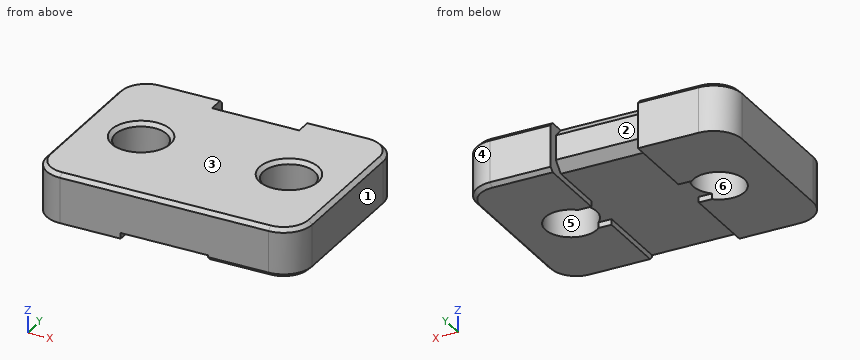
Autodesk Fusion 360 part; units mm, degrees
sketch "Sketch1" plane through (0, 0, 0) normal (0, 0, 1) x (1, 0, 0) in component "[a]_z_belt_clip_upper_x4"
  line L0 (14, -10) -> (-14, -10)
  line L1 (-14, -10) -> (-14, 10)
  line L2 (-14, 10) -> (14, 10)
  line L3 (14, 10) -> (14, -10)
  line L4 (14, -10) -> (-14, 10) construction
  line L5 (-14, -10) -> (14, 10) construction
  circle A0 centre (-7.8, 0) radius 2.7
  circle A1 centre (7.8, 0) radius 2.7
  dimension "d4" = 28
  dimension "d5" = 20
  dimension "d6" = 5.4
  dimension "d7" = 5.4
  dimension "d8" = 6.2
  dimension "d9" = 6.2
extrude "Extrude1" add sketch "Sketch1" along normal mid plane 5.2 in component "[a]_z_belt_clip_upper_x4"
fillet "Fillet1" radius 3 4 edges at (14, -10, 0) (14, 10, 0) (-14, -10, 0) (-14, 10, 0) in component "[a]_z_belt_clip_upper_x4"
sketch "Sketch2" plane through (0, 0, 2.6) normal (0, 0, 1) x (-1, 0, 0) in component "[a]_z_belt_clip_upper_x4"
  arc A0 (11, -10) -> (14, -7) centre (11, -7) ccw
  line L0 (14, -7) -> (14, 7)
  arc A1 (14, 7) -> (11, 10) centre (11, 7) ccw
  line L1 (11, 10) -> (-11, 10)
  arc A2 (-11, 10) -> (-14, 7) centre (-11, 7) ccw
  line L2 (-14, 7) -> (-14, -7)
  arc A3 (-14, -7) -> (-11, -10) centre (-11, -7) ccw
  line L3 (-11, -10) -> (11, -10)
  circle A4 centre (-7.8, 0) radius 2.7
  circle A5 centre (7.8, 0) radius 2.7
  line L4 (-4.6, -9) -> (4.6, -9)
  line L5 (4.6, -9) -> (4.6, -10)
  line L6 (4.6, -10) -> (-4.6, -10)
  line L7 (-4.6, -10) -> (-4.6, -9)
  line L8 (-4.6, -9) -> (4.6, -10) construction
  line L9 (4.6, -9) -> (-4.6, -10) construction
  line L10 (0, 0) -> (0, -20) construction
  point P0 (0, -9.5)
  dimension "d14" = 9.2
  dimension "d15" = 1
extrude "Extrude2" cut sketch "Sketch2" along normal through all and the other way through all contours L3 L4 L5 L6 L7 in component "[a]_z_belt_clip_upper_x4"
sketch "Sketch3" plane through (0, 0, -2.6) normal (0, 0, -1) x (1, 0, 0) in component "[a]_z_belt_clip_upper_x4"
  line L0 (4.6, -9) -> (4.6, -10)
  line L1 (4.6, -10) -> (11, -10)
  arc A0 (11, -10) -> (14, -7) centre (11, -7) ccw
  line L2 (14, -7) -> (14, 7)
  arc A1 (14, 7) -> (11, 10) centre (11, 7) ccw
  line L3 (11, 10) -> (-11, 10)
  arc A2 (-11, 10) -> (-14, 7) centre (-11, 7) ccw
  line L4 (-14, 7) -> (-14, -7)
  arc A3 (-14, -7) -> (-11, -10) centre (-11, -7) ccw
  line L5 (-11, -10) -> (-4.6, -10)
  line L6 (-4.6, -10) -> (-4.6, -9)
  line L7 (-4.6, -9) -> (4.6, -9)
  circle A4 centre (7.8, 0) radius 2.7
  circle A5 centre (-7.8, 0) radius 2.7
  line L8 (7.6, -2) -> (-7.6, -2)
  line L9 (-7.6, -2) -> (-7.6, 2)
  line L10 (-7.6, 2) -> (7.6, 2)
  line L11 (7.6, 2) -> (7.6, -2)
  line L12 (7.6, -2) -> (-7.6, 2) construction
  line L13 (-7.6, -2) -> (7.6, 2) construction
  line L14 (4.6, -10) -> (-4.6, -10)
  line L15 (-4.6, -10) -> (-4.6, 10)
  line L16 (-4.6, 10) -> (4.6, 10)
  line L17 (4.6, 10) -> (4.6, -10)
  line L18 (4.6, -10) -> (-4.6, 10) construction
  line L19 (-4.6, -10) -> (4.6, 10) construction
  dimension "d17" = 4
  dimension "d18" = 15.2
extrude "Extrude3" cut sketch "Sketch3" against normal blind 0.6 contours L0 L6 L7 L14 L15 L17 | L7 L8 L15 L17 | A4 L8 L10 L17 | L8 L10 L15 L17 | A5 L8 L10 L15 | A4 L8 L10 L11 | L3 L10 L15 L16 L17 | A5 L8 L9 L10 picked at (8.5667, 0) picked at (-6.7667, 0) in component "[a]_z_belt_clip_upper_x4"
chamfer "Chamfer1" distance 0.4 angle 45 16 edges at (-10.3173, 0.9764, 2.6) (5.2827, 0.9764, 2.6) (14, 0, 2.6) (13.1213, -9.1213, 2.6) (0, -10, 2.6) (-13.1213, -9.1213, 2.6) (-14, 0, 2.6) (-13.1213, 9.1213, 2.6) (-7.8, 10, 2.6) (7.8, 10, 2.6) (13.1213, 9.1213, 2.6) (7.8, -10, -2.6) (7.8, 10, -2.6) (13.1213, 9.1213, -2.6) (14, 0, -2.6) (13.1213, -9.1213, -2.6) in component "[a]_z_belt_clip_upper_x4"
chamfer "Chamfer2" distance 1 angle 45 2 edges at (0, 9, 2.6) (0, 9, -2) in component "[a]_z_belt_clip_upper_x4"
component "[a]_z_belt_clip_upper_x4" placed x (1, 0, 0) y (0, 1, 0) z (0, 0, 1) at (0, 0, 0)
equation "tolerance = 0.2 mm"
equation "chamfer = 0.4 mm"
equation "z_belt_width = 9 mm"
equation "d4 = z_belt_width + 19 mm"
equation "d10 = ( 5.2 / 2 ) * 1 mm"
equation "d14 = z_belt_width + tolerance"
equation "d18 = z_belt_width + tolerance + 6 mm"
equation "d21 = chamfer"
Read the model definition and answer for the solid it produces. Units are mm, in the model's axes. Face numbers are marked on the shaded views. A direction names the side the tool comes from. Coordinates: 2 decimals unless noted, no trailing zeros. Write each loop counter-clockwise with the first axis right and the second up, starting at its lowest first coordinate (ties: lowest second). Pieces come first, ordered by that corner, then holes. Notation, with made-up numbers: (-21.75, -6.75) - (-4.75, -6.75) arc R24 cw to (-4.75, 27.25) - close; hole circle Ø6 at (84.5, 28). An arc over 180 degrees is marked (long way). Answer as a JSON object with one key per item and string values. Group by question number.
1. Each of these flat-tipped pins is pushed along its axis until it touches: P1, Ø0.5, axis at y = -5.5, z = -2.5, coming from the +X side; P2, Ø6, axis at x = 0, y = -4.5, coming from the -Z side; P3, Ø0.5, axis at x = 5, z = -2.5, coming from the -Y side. Where does it stop, or does it pass through?
2. Consider L1, parallel to Y at x = 7.8, z = -0.35; L2, parallel to Z at x = 1.5, y = 4; L3, parallel to Y at x = 4, z = 1. Determine where each line is inside the solid, lowest interval first. Write a range as [from, to].
3. A cutting plane is placed at A-A (y = 0). Determine the outline of the cut face in (x, z), plus the area to 3 significant figures.
4. The mould has two halves that part along X. Classify the marked faces 3, 4, 5 and 6: +X half, -X half, draft (parallel to the pull), parting line (faces both ways), or undercut.
5. Which of the six approach directions +Z, -Z, +X, -X, +Y, -Y give full straight-line access (tool end or side, diameter ignored) to the marked faces 1 and 2?
6. A cutting plane is placed at D-D (x = 2.5). Determine the outline of the cut face in (y, z).
7. A cutting plane is placed at C-C (z = 0.05). Determine the outline of the cut face in (x, y).
8. A cutting plane is placed at B-B (x = 7.8). Determine the outline of the cut face in (y, z).
Worked out:
{
 "1": {"P1": "stops at x = 13.95", "P2": "stops at z = -2", "P3": "stops at y = -9.95"},
 "2": {"L1": "y = [-10, -2.7], [2.7, 10]", "L2": "z = [-2, 2.6]", "L3": "y = [-10, 9]"},
 "3": {"outline": "(-14, -2.6) - (-10.5, -2.6) - (-10.5, 2.2) - (-10.9, 2.6) - (-13.6, 2.6) - (-14, 2.2) - close; (-5.1, -2) - (5.1, -2) - (5.1, 2.2) - (4.7, 2.6) - (-4.7, 2.6) - (-5.1, 2.2) - close; (10.5, -2.6) - (13.6, -2.6) - (14, -2.2) - (14, 2.2) - (13.6, 2.6) - (10.9, 2.6) - (10.5, 2.2) - close", "area": "82.8 mm²"},
 "4": {"face 3": "draft", "face 4": "+X half", "face 5": "undercut", "face 6": "undercut"},
 "5": {"face 1": "+Z, -Z, +X, +Y, -Y", "face 2": "+Z, -Z, +Y"},
 "6": {"outline": "(-10, -2) - (8, -2) - (9, -1) - (9, 1.6) - (8, 2.6) - (-9.6, 2.6) - (-10, 2.2) - close"},
 "7": {"outline": "(-14, -7) arc R3 ccw to (-11, -10) - (11, -10) arc R3 ccw to (14, -7) - (14, 7) arc R3 ccw to (11, 10) - (4.6, 10) - (4.6, 9) - (-4.6, 9) - (-4.6, 10) - (-11, 10) arc R3 ccw to (-14, 7) - close; hole circle Ø5.4 at (-7.8, 0); hole circle Ø5.4 at (7.8, 0)"},
 "8": {"outline": "(-10, -2.2) - (-9.6, -2.6) - (-2.7, -2.6) - (-2.7, 2.2) - (-3.1, 2.6) - (-9.6, 2.6) - (-10, 2.2) - close; (2.7, -2.6) - (9.6, -2.6) - (10, -2.2) - (10, 2.2) - (9.6, 2.6) - (3.1, 2.6) - (2.7, 2.2) - close"}
}
